The model under review builds one solid part; all positions refer to its coordinate system, in mm. A direction names the side the tool comes from. Coordinates: 2 decimals unless noted, no trailing zeros. Loops run counter-clockwise (first coordinate to the right, second up) from the corner with the lowest first, then second, coordinate; pieces in that order, holes last. Notation, with made-up numbers: M 68.5,58.25 L 95.5,58.25 A18 cw 95.5,63.25 Z; hole C 19.25,54.5 d8. An arc over 180 degrees is marked long. Return JSON: item names as keys, results as strings.
Autodesk Inventor part; units mm, degrees
ref_plane "YZ Plane" through (0, 0, 0) normal (1, 0, 0) x (0, 1, 0)
ref_plane "XZ Plane" through (0, 0, 0) normal (0, 1, 0) x (-1, 0, 0)
ref_plane "XY Plane" through (0, 0, 0) normal (0, 0, 1) x (1, 0, 0)
sketch "Sketch1" plane through (0, 0, 0) normal (0, 0, 1) x (1, 0, 0)
  circle A0 centre (0, 0) radius 2.5
  circle A1 centre (-5, 0) radius 1.5
  arc A2 (-5.9, 2.8618) -> (-5.9, -2.8618) centre (-5, 0) ccw
  arc A3 (-1.35, -4.2927) -> (-1.35, 4.2927) centre (0, 0) ccw
  line L0 (-5.9, 2.8618) -> (-1.35, 4.2927)
  line L1 (-5.9, -2.8618) -> (-1.35, -4.2927)
  dimension "d0" = 5
  dimension "d1" = 3
  dimension "d2" = 9
  dimension "d3" = 5
  dimension "d4" = 1.5
extrude "Extrusion1" add sketch "Sketch1" along normal blind 8
sketch "Sketch2" plane through (0, 0, 0) normal (0, 0, -1) x (-1, 0, 0)
  circle A0 centre (5, 0) radius 1.5
  circle A1 centre (5, 0) radius 1
  point P0 (0, 0)
  dimension "d21" = 2
extrude "Extrusion2" add sketch "Sketch2" against normal blind 2
sketch "Sketch3" plane through (0, 0, 0) normal (1, 0, 0) x (0, 1, 0)
  circle A0 centre (0, 4) radius 1.5
  line L0 (2.5, 8) -> (2.5, 0)
  point P0 (0, 0)
  point P1 (2.5, 4)
  dimension "d13" = 3
properties part number "Anode Holding Nut" material "Stainless Steel"
1. Add section C-C on z = 3.75. Give the boundary of the cut face in (x, y), plus the area to 3 significant figures.
Check values:
{"outline": "M -5.9,-2.86 L -1.35,-4.29 A4.5 ccw long -1.35,4.29 L -5.9,2.86 A3 ccw Z; hole C -5,0 d3; hole C 0,0 d5", "area": "58.4 mm²"}
2. Add section D-D on x = -5. Give the boundary of the cut face in (y, z), plus the area to 3 significant figures.
Check values:
{"outline": "M -3.14,0 L -1,0 L -1,2 L -1.5,2 L -1.5,8 L -3.14,8 Z; M 1,0 L 3.14,0 L 3.14,8 L 1.5,8 L 1.5,2 L 1,2 Z", "area": "28.3 mm²"}
3. Add section A-A on x = 0. Give the boundary of the cut face in (y, z).
Check values:
{"outline": "M -4.5,0 L -2.5,0 L -2.5,8 L -4.5,8 Z; M 2.5,0 L 4.5,0 L 4.5,8 L 2.5,8 Z"}
4. Insertion check: pin 1 Ø4 at (x, z) = (-4.5, 1) entering from -Y; pin 2 Ø1.2 at (x, y) = (-5, 0) entering from -Z; pin 3 Ø1.5 at (y, z) = (1, 6) entering from -X; pin 4 Ø3 at (x, z) = (-5, 7) entering from -Y. Each pin has a flat end and moves straight along its axis. Give the tip position at first contact, or say it passes through.
Check values:
{"pin 1": "y = -3.93", "pin 2": "through", "pin 3": "x = -7.99", "pin 4": "y = -3.62"}
5. To check wall thickness, follow line 1 (X direction, y = -0.75, z = 2.75); line 2 (Y direction, x = 0, z = 2.75); line 3 (X direction, y = -0.25, z = 6.75). State the ranges of each line that lie inside material, in increasing order.
Check values:
{"line 1": "-7.9 to -6.3, -3.7 to -2.38, 2.38 to 4.44", "line 2": "-4.5 to -2.5, 2.5 to 4.5", "line 3": "-7.99 to -6.48, -3.52 to -2.49, 2.49 to 4.49"}
6. Machinability: for faces 1 (the face through (-6.2, 0.9, 5)), 2 (the face through (-8, 0, 4)), which of the approach directions +Z, -Z, +X, -X, +Y, -Y give a long, thin tool a straight path to every point of the face, cutting with its end or side? Answer none if there is none.
Check values:
{"face 1": "+Z", "face 2": "+Z, -Z, -X"}
7. The part is to be moulded in two halves that separate along Y. For faces 3 (the face through (-0.54, 2.44, 3.94)), 4 (the face through (-3, 0, 8)), 5 (the face through (-3.657, 3.567, 3.944)), say which applies: released by +Y, released by -Y, zero draft, split by the parting line, or undercut.
Check values:
{"face 3": "undercut", "face 4": "zero draft", "face 5": "released by +Y"}
8. Add section B-B on y = 0. Give the boundary of the cut face in (x, z), plus the area to 3 significant figures.
Check values:
{"outline": "M -8,0 L -6,0 L -6,2 L -6.5,2 L -6.5,8 L -8,8 Z; M -4,0 L -2.5,0 L -2.5,8 L -3.5,8 L -3.5,2 L -4,2 Z; M 2.5,0 L 4.5,0 L 4.5,8 L 2.5,8 Z", "area": "38.0 mm²"}
